from build123d import *

# Parameters (mm, degrees)
RESSALTO_EXTRUS_O1_DEPTH        = 128.2
FURO_ROSCADO_DE_M61_D           = 5
FURO_ROSCADO_DE_M61_DEPTH       = 20.45
FURO_ROSCADO_DE_M61_CSINK_D     = 6.05
FURO_ROSCADO_DE_M61_CSINK_ANGLE = 90
FURO_ROSCADO_DE_M61_TIP         = 1.502151548
ESBO_O4_R                       = 12.5
CORTE_EXTRUS_O1_DEPTH           = 157.956172227
ESBO_O5_R                       = 29
CORTE_EXTRUS_O2_DEPTH           = 50
ESBO_O6_R                       = 20
CORTE_EXTRUS_O3_DEPTH           = 70


with BuildPart() as part:
    # Esboço1 → Ressalto-extrusão1 (new body)
    with BuildSketch(Plane(origin=(0, 0, 0), x_dir=(0, 0, -1), z_dir=(1, 0, 0))):
        Polygon((0, 49), (16.5, 66), (45.5, 66), (62, 49), (62, 0), (0, 0), align=None)
    extrude(amount=-RESSALTO_EXTRUS_O1_DEPTH)

    # Furo roscado de M61
    with Locations(Plane(origin=(0, 0, 0), x_dir=(0, 0, -1), z_dir=(1, 0, 0))):
        with Locations((13.5, 52), (48.5, 52), (48.5, 17), (13.5, 17)):
            CounterSinkHole(FURO_ROSCADO_DE_M61_D / 2, FURO_ROSCADO_DE_M61_CSINK_D / 2, depth=FURO_ROSCADO_DE_M61_DEPTH, counter_sink_angle=FURO_ROSCADO_DE_M61_CSINK_ANGLE)
            with Locations((0, 0, -(FURO_ROSCADO_DE_M61_DEPTH + FURO_ROSCADO_DE_M61_TIP / 2))):  # 118° drill point
                Cone(0, FURO_ROSCADO_DE_M61_D / 2, FURO_ROSCADO_DE_M61_TIP, mode=Mode.SUBTRACT)

    # Esboço4 → Corte-extrusão1 (cut, through all)
    with BuildSketch(Plane(origin=(0, 0, 0), x_dir=(0, 0, -1), z_dir=(1, 0, 0))):
        with Locations((31, 34.5)):
            Circle(ESBO_O4_R)
    extrude(amount=-CORTE_EXTRUS_O1_DEPTH, mode=Mode.SUBTRACT)

    # Esboço5 → Corte-extrusão2 (cut)
    with BuildSketch(Plane.ZY.offset(128.2)):
        with Locations((-31, 34.5)):
            Circle(ESBO_O5_R)
    extrude(amount=-CORTE_EXTRUS_O2_DEPTH, mode=Mode.SUBTRACT)

    # Esboço6 → Corte-extrusão3 (cut)
    with BuildSketch(Plane(origin=(0, 0, 0), x_dir=(0, 0, -1), z_dir=(1, 0, 0))):
        with Locations((31, 34.5)):
            Circle(ESBO_O6_R)
    extrude(amount=-CORTE_EXTRUS_O3_DEPTH, mode=Mode.SUBTRACT)


solid = part.part
Verification items for the finished model (mm, model axes). A direction names the side the tool comes from. Round coordinates to 2 decimals unless told otherwise and drop trailing zeros. Write each loop counter-clockwise with the first axis right and the second up, starting at its lowest first coordinate (ties: lowest second). Pieces come first, ordered by that corner, then holes.
(1) Depth check by flat-ended pin: pin 1 Ø1.5 at (y, z) = (59, -15) entering from +X; pin 2 Ø12 at (y, z) = (41, -38.5) entering from +X; pin 3 Ø3 at (y, z) = (52, -13.5) entering from -X; pin 4 Ø3 at (x, z) = (-52.5, -48) entering from +Y. Enter the tip coordinate at first touch or a pass-through.
Returned:
pin 1: stops at x = 0
pin 2: stops at x = -70
pin 3: stops at x = -78.2
pin 4: stops at y = 64.97
(2) Access from +Z, -Z, +X, -X, +Y, -Y to the whole of each face (thin tool, end or side, straight path). Record for faces 1 (the flat face through (-63, 66, -31)), 2 (the flat face through (-70, 44, -40)).
Returned:
face 1: +Z, -Z, +X, -X, +Y
face 2: +X
(3) Section check B-B (x = -11). Enter the section's corners in (y, z).
Returned:
outline: (0, -62) - (49, -62) - (66, -45.5) - (66, -16.5) - (49, 0) - (0, 0) - close; hole circle Ø5 at (17, -48.5); hole circle Ø40 at (34.5, -31); hole circle Ø5 at (17, -13.5); hole circle Ø5 at (52, -48.5); hole circle Ø5 at (52, -13.5)
(4) Mould release check, pull along Y, two halves, no side actions. Record for faces 3 (the flat face through (-63.203, 57.381, -8.135)), 4 (the flat face through (-63, 0, -31)), 5 (the cylindrical face through (-103.55, 63.253, -34.775)): pulls with the +Y half, pulls with the -Y half, needs draft (parallel to the pull), parting line crosses it, or undercut.
Returned:
face 3: pulls with the +Y half
face 4: pulls with the -Y half
face 5: undercut
(5) Section check D-D (x = -32). Enter the section's corners in (y, z), plus the area to 3 significant figures.
Returned:
outline: (0, -62) - (49, -62) - (66, -45.5) - (66, -16.5) - (49, 0) - (0, 0) - close; hole circle Ø40 at (34.5, -31)
area: 2,550 mm2
(6) Section check A-A (y = 34.5). Enter the section's corners in (x, z), plus the area to 3 significant figures.
Returned:
outline: (-128.2, -62) - (0, -62) - (0, -51) - (-70, -51) - (-70, -43.5) - (-78.2, -43.5) - (-78.2, -60) - (-128.2, -60) - close; (-128.2, -2) - (-78.2, -2) - (-78.2, -18.5) - (-70, -18.5) - (-70, -11) - (0, -11) - (0, 0) - (-128.2, 0) - close
area: 2,040 mm2
(7) Material ranges on line 1 (Z direction, x = -13, y = 17); line 2 (Y direction, x = -74.25, z = -31); line 3 (Y direction, x = -6.25, z = -13.5), recorded low to high.
Returned:
line 1: z = -62 to -51, -46 to -40.68, -21.32 to -16, -11 to 0
line 2: y = 0 to 22, 47 to 66
line 3: y = 0 to 14.5, 19.5 to 24.82, 44.18 to 49.5, 54.5 to 62.91
(8) Section check C-C (z = -38.5). Enter the section's corners in (x, y), plus the area to 3 significant figures.
Returned:
outline: (-128.2, 0) - (0, 0) - (0, 15.96) - (-70, 15.96) - (-70, 24.5) - (-78.2, 24.5) - (-78.2, 6.49) - (-128.2, 6.49) - close; (-128.2, 62.51) - (-78.2, 62.51) - (-78.2, 44.5) - (-70, 44.5) - (-70, 53.04) - (0, 53.04) - (0, 66) - (-128.2, 66) - close
area: 2,900 mm2
